Check sheet for the modelled part. Datum: model origin and axes. Units: mm. A direction names the side the tool comes from. Round coordinates to 2 decimals unless told otherwise and drop trailing zeros. Write each loop counter-clockwise with the first axis right and the second up, starting at its lowest first coordinate (ties: lowest second). Pieces come first, ordered by that corner, then holes. Notation, with made-up numbers: (41, 0.25) - (83, 0.25) arc R21 ccw to (83, 29.25) - close; hole circle Ø8 at (67.25, 41.25). An arc over 180 degrees is marked (long way). Answer as a JSON object with one key per item and string values. Group by question number.
Item 1: Gauge pin test, flat ends, axial feed: P1, Ø5, axis at x = 23, z = 51.5, coming from the -Y side; P2, Ø1.5, axis at y = 6.5, z = 23.5, coming from the -X side; P3, Ø1.5, axis at y = -23.5, z = 58, coming from the -X side; P4, Ø4, axis at x = 8.1, y = 0, coming from the -Z side. Record the tip position at first contact, or that the pin passes through.
Item 2: Sectioned sample at B-B on y = 0. Count the separate pieces of the cut face and the enclosed holes in it, plus the area to 3 significant figures.
Item 3: Thickness scan on line 1 (Z direction, x = -5, y = 10); line 2 (X direction, y = -7, z = 39); line 3 (X direction, y = -13, z = 32). Record the ranges inside material, lowest first.
Item 4: Set-up check for faces 1 (the cylindrical face through (-31.22, 1.37, 1.48)), 2 (the cylindrical face through (0, -2, 65)), 3 (the cylindrical face through (7.123, 11.172, 75.07)): record each of +Z, -Z, +X, -X, +Y, -Y from which the full face is reachable in a straight line by a thin tool's end or side.
Item 5: Sectioned sample at A-A on z = 28. Record the boundary of the cut face in (x, y), plus the area to 3 significant figures.
Item 6: Release check for a two-part mould opening along Y. For faces 4 (the flat face through (-17, 27, 8)), 5 (the cylindrical face through (5.6, 0.1, 65.1)), 6 (the conical face through (12.98, -5.38, 79.2)) record: pulls with the +Y half, pulls with the -Y half, needs draft (parallel to the pull), parting line crosses it, or undercut.
```python
from build123d import *

# Parameters (mm, degrees)
SKETCH1_R           = 31.25
BOSS_EXTRUDE1_DEPTH = 80
SKETCH2_R           = 32.5
BOSS_EXTRUDE2_DEPTH = 5
CHAMFER1_SIZE       = 18
FILLET2_R           = 5
SKETCH6_R           = 13.25
CUT_EXTRUDE3_DEPTH  = 10
SKETCH7_R           = 28.75
CUT_EXTRUDE4_DEPTH  = 60
SKETCH8_R           = 2
SKETCH8_R_2         = 2.5
CUT_EXTRUDE5_DEPTH  = 84.740671122


with BuildPart() as part:
    # Sketch1 → Boss-Extrude1 (new body)
    with BuildSketch(Plane.XY):
        Circle(SKETCH1_R)
    extrude(amount=BOSS_EXTRUDE1_DEPTH)

    # Sketch2 → Boss-Extrude2 (add)
    with BuildSketch(Plane.XY.offset(3)):
        Circle(SKETCH2_R)
    extrude(amount=BOSS_EXTRUDE2_DEPTH)

    # Chamfer1
    chamfer1_edges = [part.edges().sort_by_distance(p)[0] for p in [
        (-31.25, 0, 80),
    ]]
    chamfer(chamfer1_edges, length=CHAMFER1_SIZE)

    # Fillet2
    fillet2_edges = [part.edges().sort_by_distance(p)[0] for p in [
        (-31.25, 0, 62),
    ]]
    fillet(fillet2_edges, radius=FILLET2_R)

    # Sketch6 → Cut-Extrude3 (cut)
    with BuildSketch(Plane.XY.offset(80)):
        Circle(SKETCH6_R)
    extrude(amount=-CUT_EXTRUDE3_DEPTH, mode=Mode.SUBTRACT)

    # Sketch7 → Cut-Extrude4 (cut)
    with BuildSketch(Plane(origin=(0, 0, 0), x_dir=(-1, 0, 0), z_dir=(0, 0, -1))):
        Circle(SKETCH7_R)
    extrude(amount=-CUT_EXTRUDE4_DEPTH, mode=Mode.SUBTRACT)

    # Sketch8 → Cut-Extrude5 (cut, through all)
    with BuildSketch(Plane.XY.offset(70)):
        Circle(SKETCH8_R)
        with Locations((8.096346775, 0)):
            Circle(SKETCH8_R_2)
    extrude(amount=-CUT_EXTRUDE5_DEPTH, mode=Mode.SUBTRACT)


solid = part.part
```
Completed:
{
 "1": {"P1": "y = -23.59", "P2": "x = -30.72", "P3": "x = -21.42", "P4": "through"},
 "2": {"separate pieces": "3", "enclosed holes": "0", "area": "882 mm²"},
 "3": {"line 1": "60 to 70", "line 2": "-30.46 to -27.88, 27.88 to 30.46", "line 3": "-28.42 to -25.64, 25.64 to 28.42"},
 "4": {"face 1": "-Z", "face 2": "+Z, -Z", "face 3": "+Z"},
 "5": {"outline": "circle Ø62.5 at (0, 0); hole circle Ø57.5 at (0, 0)", "area": "471 mm²"},
 "6": {"face 4": "needs draft", "face 5": "undercut", "face 6": "parting line crosses it"}
}
